from build123d import *

# Parameters (mm, degrees)
SKETCH1_W           = 100
SKETCH1_H           = 300
BOSS_EXTRUDE1_DEPTH = 2
SKETCH2_R           = 1
CUT_EXTRUDE1_DEPTH  = 10
SKETCH3_R           = 15
CUT_EXTRUDE2_DEPTH  = 10
SKETCH4_R           = 1
CUT_EXTRUDE3_DEPTH  = 10


with BuildPart() as part:
    # Sketch1 → Boss-Extrude1 (new body)
    with BuildSketch(Plane.XY):
        Rectangle(SKETCH1_W, SKETCH1_H)
    extrude(amount=BOSS_EXTRUDE1_DEPTH)

    # Sketch2 → Cut-Extrude1 (cut)
    with BuildSketch(Plane.XY.offset(2)):
        with Locations((-39, 122)):
            Circle(SKETCH2_R)
        with Locations((-39, 77)):
            Circle(SKETCH2_R)
        with Locations((39, 122)):
            Circle(SKETCH2_R)
        with Locations((39, 77)):
            Circle(SKETCH2_R)
        with Locations((-39, 21)):
            Circle(SKETCH2_R)
        with Locations((-39, -24)):
            Circle(SKETCH2_R)
        with Locations((39, 21)):
            Circle(SKETCH2_R)
        with Locations((39, -24)):
            Circle(SKETCH2_R)
        with Locations((-39, -80)):
            Circle(SKETCH2_R)
        with Locations((-39, -125)):
            Circle(SKETCH2_R)
        with Locations((39, -80)):
            Circle(SKETCH2_R)
        with Locations((39, -125)):
            Circle(SKETCH2_R)
    extrude(amount=-CUT_EXTRUDE1_DEPTH, mode=Mode.SUBTRACT)

    # Sketch3 → Cut-Extrude2 (cut)
    with BuildSketch(Plane(origin=(0, 0, 0), x_dir=(-1, 0, 0), z_dir=(0, 0, -1))):
        with Locations((0, 91)):
            Circle(SKETCH3_R)
    extrude(amount=-CUT_EXTRUDE2_DEPTH, mode=Mode.SUBTRACT)

    # Sketch4 → Cut-Extrude3 (cut)
    with BuildSketch(Plane(origin=(0, 0, 0), x_dir=(-1, 0, 0), z_dir=(0, 0, -1))):
        with Locations((-26.5, 139.5)):
            Circle(SKETCH4_R)
        with Locations((26.5, 139.5)):
            Circle(SKETCH4_R)
        with Locations((-26.5, -140.5)):
            Circle(SKETCH4_R)
        with Locations((26.5, -140.5)):
            Circle(SKETCH4_R)
    extrude(amount=-CUT_EXTRUDE3_DEPTH, mode=Mode.SUBTRACT)


solid = part.part
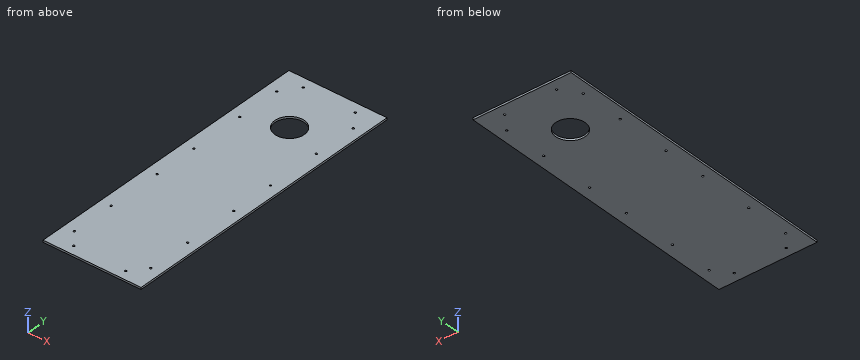
Part model, mm, in its own coordinate system. Coordinates: 2 decimals unless noted, no trailing zeros. Write each loop counter-clockwise with the first axis right and the second up, starting at its lowest first coordinate (ties: lowest second). Pieces come first, ordered by that corner, then holes. Notation, with made-up numbers: (-0.5, 26) - (52.5, 26) arc R34 cw to (52.5, 65) - close; hole circle Ø10 at (-24.5, 41). An arc over 180 degrees is marked (long way). Put each result on its own line as item: value.
1. Band-saw the part on A-A (x = -9.5). Write the cut outline in (y, z), then the cut area to 3 significant figures.
Final values:
outline: (-150, 0) - (79.39, 0) - (79.39, 2) - (-150, 2) - close; (102.61, 0) - (150, 0) - (150, 2) - (102.61, 2) - close
area: 554 mm²
2. Band-saw the part on B-B (z = 0.3). Give the number of separate pieces and of enclosed holes in the cut face, then the cut area to 3 significant figures.
Final values:
separate pieces: 1
enclosed holes: 17
area: 29,200 mm²
3. Probe line 1 along X through (y, z) = (-80, 1.4); line 2 along Y through (x, z) = (-26.5, 1.45); line 3 along Y through (x, z) = (-12.5, 0.2). List the from-to ranges inside material, lowest first. Write a range as [from, to].
Final values:
line 1: x = [-50, -40], [-38, 38], [40, 50]
line 2: y = [-150, -141.5], [-139.5, 138.5], [140.5, 150]
line 3: y = [-150, 82.71], [99.29, 150]
4. Flat gauge pin, fed straight in: pin 1 Ø1.6 at (x, y) = (-39, -125) entering from -Z. Where does the tip first touch, or does it go through?
Final values:
pin 1: passes through
